Autodesk Inventor part; units mm, degrees
ref_plane "dia1_XY" through (0, 3.175, 0) normal (1, 0, 0) x (0, 0, -1)
ref_plane "dia1_YZ" through (0, 3.175, 0) normal (0, 0, -1) x (0, 1, 0)
ref_plane "dia1_ZX" through (0, 3.175, 0) normal (0, 1, 0) x (1, 0, 0)
sketch "Sketch_1" plane through (0, 0, 0) normal (0, 0, 1) x (1, 0, 0)
  line L0 (97.7646, 0) -> (0, 0)
  line L1 (0, 0) -> (0, 3.175)
  line L2 (0, 3.175) -> (60.325, 3.175)
  line L3 (60.325, 3.175) -> (60.325, 9.6202)
  line L4 (60.325, 9.6202) -> (97.7646, 9.6202)
  line L5 (97.7646, 9.6202) -> (97.7646, 0)
  line L6 (97.7646, 0) -> (0, 0)
revolve "Revolution1" add sketch "Sketch_1" angle 360 about axis through (97.7646, 0, 0) along (1, 0, 0)
sketch "Sketch_3" plane through (0, 0, 0) normal (0, 0, 1) x (1, 0, 0)
  line L0 (0, 0) -> (-12.7, 0)
  line L1 (-12.7, 0) -> (-12.7, 2.634)
  line L2 (-12.7, 2.634) -> (-12.159, 3.175)
  line L3 (-12.159, 3.175) -> (0, 3.175)
  line L4 (0, 3.175) -> (0, 0)
  line L5 (0, 0) -> (-12.7, 0)
revolve "Revolution2" add sketch "Sketch_3" angle 360 about axis through (0, 0, 0) along (1, 0, 0)
sketch "Sketch_30" plane through (0, 0, 0) normal (0, 0, 1) x (1, 0, 0)
  line L0 (0, 0) -> (-0.254, 0)
  line L1 (-0.254, 2.921) -> (0, 2.921)
  line L2 (0, 2.921) -> (0, 3.429)
  line L3 (0, 3.429) -> (-0.254, 3.429)
  line L4 (-0.254, 3.429) -> (-0.254, 2.921)
revolve "Revolution3" cut sketch "Sketch_30" angle 360 about axis through (0, 0, 0) along (1, 0, 0)
ref_plane "dia1_XY" through (0, 3.175, 0) normal (1, 0, 0) x (0, 0, -1)
ref_plane "dia1_YZ" through (0, 3.175, 0) normal (0, 0, -1) x (0, 1, 0)
ref_plane "dia1_ZX" through (0, 3.175, 0) normal (0, 1, 0) x (1, 0, 0)
ref_plane "dia12_XY" through (0, 0, 10.2235) normal (1, 0, 0) x (0, 0, -1)
ref_plane "dia12_YZ" through (0, 0, 10.2235) normal (0, 0, -1) x (0, 1, 0)
ref_plane "dia12_ZX" through (0, 0, 10.2235) normal (0, 1, 0) x (1, 0, 0)
ref_plane "dia2_XY" through (0, -3.175, 0) normal (1, 0, 0) x (0, 0, -1)
ref_plane "dia2_YZ" through (0, -3.175, 0) normal (0, 0, -1) x (0, 1, 0)
ref_plane "dia2_ZX" through (0, -3.175, 0) normal (0, 1, 0) x (1, 0, 0)
ref_plane "dia22_XY" through (0, 0, -10.2235) normal (1, 0, 0) x (0, 0, -1)
ref_plane "dia22_YZ" through (0, 0, -10.2235) normal (0, 0, -1) x (0, 1, 0)
ref_plane "dia22_ZX" through (0, 0, -10.2235) normal (0, 1, 0) x (1, 0, 0)
ref_plane "rl1_XY" through (-12.7, 0, 0) normal (1, 0, 0) x (0, 0, -1)
ref_plane "rl1_YZ" through (-12.7, 0, 0) normal (0, 0, -1) x (0, 1, 0)
ref_plane "rl1_ZX" through (-12.7, 0, 0) normal (0, 1, 0) x (1, 0, 0)
ref_plane "rl2_XY" through (0, 0, 0) normal (1, 0, 0) x (0, 0, -1)
ref_plane "rl2_YZ" through (0, 0, 0) normal (0, 0, -1) x (0, 1, 0)
ref_plane "rl2_ZX" through (0, 0, 0) normal (0, 1, 0) x (1, 0, 0)
ref_plane "rod_cp_XY" through (0, 0, 0) normal (1, 0, 0) x (0, 0, -1)
ref_plane "rod_cp_YZ" through (0, 0, 0) normal (0, 0, -1) x (0, 1, 0)
ref_plane "rod_cp_ZX" through (0, 0, 0) normal (0, 1, 0) x (1, 0, 0)
ref_plane "thd1_XY" through (-12.7, 3.175, 0) normal (1, 0, 0) x (0, 0, -1)
ref_plane "thd1_YZ" through (-12.7, 3.175, 0) normal (0, 0, -1) x (0, 1, 0)
ref_plane "thd1_ZX" through (-12.7, 3.175, 0) normal (0, 1, 0) x (1, 0, 0)
ref_plane "thd2_XY" through (-12.7, -3.175, 0) normal (1, 0, 0) x (0, 0, -1)
ref_plane "thd2_YZ" through (-12.7, -3.175, 0) normal (0, 0, -1) x (0, 1, 0)
ref_plane "thd2_ZX" through (-12.7, -3.175, 0) normal (0, 1, 0) x (1, 0, 0)
ref_plane "to_rod_clevis_XY" through (-16.764, 0, 0) normal (1, 0, 0) x (0, 0, -1)
ref_plane "to_rod_clevis_YZ" through (-16.764, 0, 0) normal (0, 0, -1) x (0, 1, 0)
ref_plane "to_rod_clevis_ZX" through (-16.764, 0, 0) normal (0, 1, 0) x (1, 0, 0)
properties part number "C-041.50000_rod"
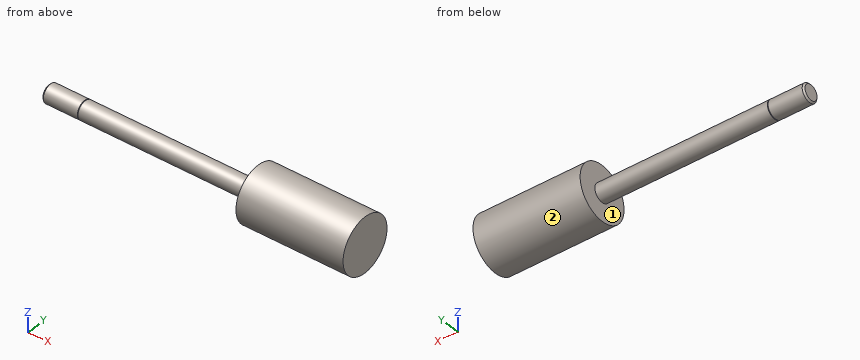
Build history of the part. All positions in model axes, mm. Face numbers are marked on the shaded views. A direction names the side the tool comes from. Give positions to 0.01 mm unless a question says otherwise; leave off trailing zeros. Loops run counter-clockwise (first coordinate to the right, second up) from the corner with the lowest first, then second, coordinate; pieces in that order, holes last.
Item 1: Slice it at A-A, the plane z = 0. List the corners of the cut face in (x, y) (3 decimals).
Answers follow:
outline: (-12.7, -2.634) - (-12.159, -3.175) - (-0.254, -3.175) - (-0.254, -2.921) - (0, -2.921) - (0, -3.175) - (60.325, -3.175) - (60.325, -9.62) - (97.765, -9.62) - (97.765, 9.62) - (60.325, 9.62) - (60.325, 3.175) - (0, 3.175) - (0, 2.921) - (-0.254, 2.921) - (-0.254, 3.175) - (-12.159, 3.175) - (-12.7, 2.634) - close
Item 2: Flat gauge pins, fed straight in: pin 1 (4 mm diameter, centred on x = 25, y = 2.5, fed in from -Z); pin 2 (1.5 mm diameter, centred on x = 1, z = -4.5, fed in from -Y); pin 3 (6 mm diameter, centred on x = 12.5, z = 4.5, fed in from +Y); pin 4 (10 mm diameter, centred on x = 39, y = 2.5, fed in from -Z) (3 decimals). Where does each tip first touch, or does it go through?
Answers follow:
pin 1: stops at z = -3.14
pin 2: passes through
pin 3: stops at y = 2.8
pin 4: stops at z = -3.175
Item 3: Slice it at C-C, the plane x = 57.5. List the corners of the cut face in (y, z) (3 decimals), and give its area (3 significant figures).
Answers follow:
outline: circle Ø6.35 at (0, 0)
area: 31.7 mm2
Item 4: Which spindle directions (+Z, -Z, +X, -X, +Y, -Y) get a long thin tool onto all of the face, cutting with end or side? Do the marked faces 1 and 2. Say none if no direction does.
Answers follow:
face 1: -X
face 2: +X, -X
Item 5: Drill centre lines: line 1 (X direction, y = -5.75, z = -2) (3 decimals); line 2 (Z direction, x = 55, y = -1.25); line 3 (Z direction, x = 63, y = 6). Where is each one in solid material? Low to high.
Answers follow:
line 1: x = 60.325 to 97.765
line 2: z = -2.92 to 2.92
line 3: z = -7.52 to 7.52
Item 6: Slice it at D-D, the plane y = -6.5. List the corners of the cut face in (x, z) (3 decimals), and give its area (3 significant figures).
Answers follow:
outline: (60.325, -7.092) - (97.765, -7.092) - (97.765, 7.092) - (60.325, 7.092) - close
area: 531 mm2
